Model file for the job. Use its own axes, mm. Face numbers are marked on the shaded views. A direction names the side the tool comes from. Give positions to 0.01 mm unless a question says otherwise; leave off trailing zeros. Loops run counter-clockwise (first coordinate to the right, second up) from the corner with the lowest first, then second, coordinate; pieces in that order, holes last. Notation, with made-up numbers: M 64,-3 L 116,-3 A17 cw 116,27 Z; hole C 76,55.25 d11. An arc over 180 degrees is marked long. Answer in a Markdown table with one row per item.
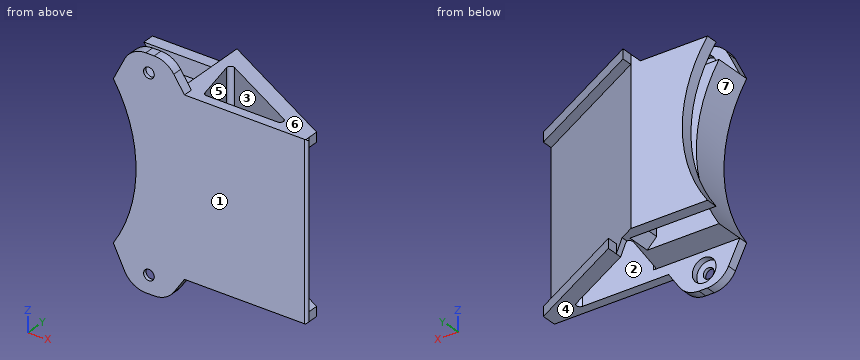
```python
from build123d import *

# Parameters (mm, degrees)
ESTRUSIONE_ESTRUSIONE1_DEPTH                         = 90
TAGLIO_ESTRUSIONE1_DEPTH                             = 60
SCHIZZO3_R                                           = 60
TAGLIO_ESTRUSIONE2_DEPTH                             = 21
ESTRUSIONE_ESTRUSIONE2_DEPTH                         = 4
FORO_LAMATO_PER_VITE_M4_A_TESTA_CILINDRI_D           = 4.5
FORO_LAMATO_PER_VITE_M4_A_TESTA_CILINDRI_DEPTH       = 8
FORO_LAMATO_PER_VITE_M4_A_TESTA_CILINDRI_CBORE_D     = 10
FORO_LAMATO_PER_VITE_M4_A_TESTA_CILINDRI_CBORE_DEPTH = 2.6
FORO_LAMATO_PER_VITE_M4_A_TESTA_CILINDRI_TIP         = 1.351936393
RACCORDO3_R                                          = 10
ESTRUSIONE_ESTRUSIONE3_DEPTH                         = 4
ESTRUSIONE_ESTRUSIONE4_DEPTH                         = 4
TAGLIO_ESTRUSIONE3_DEPTH                             = 179
SMUSSO1_SIZE                                         = 4
RACCORDO4_START                                      = -5
RACCORDO4_DEPTH                                      = 75
RACCORDO4_2_DEPTH                                    = 65
SMUSSO2_SIZE                                         = 4
SMUSSO3_SIZE                                         = 4


with BuildPart() as part:
    # Schizzo1 → Estrusione-Estrusione1 (new body)
    with BuildSketch(Plane.XY):
        Polygon((-115, 26), (0, 26), (0, 16), (-45, 16), (-45, 0), (58.302520426, 0), (0, 31), (-115, 31), align=None)
    extrude(amount=ESTRUSIONE_ESTRUSIONE1_DEPTH)

    # Schizzo2 → Taglio-Estrusione1 (cut)
    with BuildSketch(Plane(origin=(0, 31, 0), x_dir=(1, 0, 0), z_dir=(0, 1, 0))):
        with BuildLine():
            Line((-32.326881201, -65), (58.302520426, -65))
            Line((58.302520426, -65), (58.302520426, -90))
            Line((58.302520426, -90), (-115, -90))
            Line((-115, -90), (-115, 0))
            Line((-115, 0), (-32.326881201, 0))
            ThreePointArc((-32.326881201, 0), (-21.697479574, -32.5), (-32.326881201, -65))
        make_face()
    extrude(amount=-TAGLIO_ESTRUSIONE1_DEPTH, mode=Mode.SUBTRACT)

    # Schizzo3 → Taglio-Estrusione2 (cut)
    with BuildSketch(Plane.XZ):
        with Locations((-76.697479574, 32.5)):
            Circle(SCHIZZO3_R)
    extrude(amount=-TAGLIO_ESTRUSIONE2_DEPTH, mode=Mode.SUBTRACT)

    # Schizzo4 → Estrusione-Estrusione2 (add)
    with BuildSketch(Plane.XZ):
        Polygon((-26.26187707, 65), (-18.76187707, 80), (-3.76187707, 80), (3.73812293, 69), (3.73812293, 65), align=None)
        Polygon((-26.26187707, 0), (-18.76187707, -15), (-3.76187707, -15), (3.73812293, -4), (3.73812293, 0), align=None)
    extrude(amount=-ESTRUSIONE_ESTRUSIONE2_DEPTH)

    # Foro lamato per Vite M4 a testa cilindrica piana-1
    with Locations(Plane(origin=(-11.26187707, 4, 72.5), x_dir=(0, 0, 1), z_dir=(0, 1, 0))):
        with Locations((0, 0), (-80, 0)):
            CounterBoreHole(FORO_LAMATO_PER_VITE_M4_A_TESTA_CILINDRI_D / 2, FORO_LAMATO_PER_VITE_M4_A_TESTA_CILINDRI_CBORE_D / 2, FORO_LAMATO_PER_VITE_M4_A_TESTA_CILINDRI_CBORE_DEPTH, depth=FORO_LAMATO_PER_VITE_M4_A_TESTA_CILINDRI_DEPTH)
            with Locations((0, 0, -(FORO_LAMATO_PER_VITE_M4_A_TESTA_CILINDRI_DEPTH + FORO_LAMATO_PER_VITE_M4_A_TESTA_CILINDRI_TIP / 2))):  # 118° drill point
                Cone(0, FORO_LAMATO_PER_VITE_M4_A_TESTA_CILINDRI_D / 2, FORO_LAMATO_PER_VITE_M4_A_TESTA_CILINDRI_TIP, mode=Mode.SUBTRACT)

    # Raccordo3
    raccordo3_edges = [part.edges().sort_by_distance(p)[0] for p in [
        (-18.76187707, 2, 80),
        (-3.76187707, 2, 80),
        (-3.76187707, 2, -15),
        (-18.76187707, 2, -15),
    ]]
    fillet(raccordo3_edges, radius=RACCORDO3_R)

    # Schizzo9 → Estrusione-Estrusione3 (add)
    with BuildSketch(Plane.XY.offset(65)):
        Polygon((3.73812293, 0), (3.73812293, 4), (0, 4), (0, 35.530280203), (54.802520426, 6.391263214), (54.802520426, 0), align=None)
    extrude(amount=ESTRUSIONE_ESTRUSIONE3_DEPTH)

    # Schizzo10 → Estrusione-Estrusione4 (add)
    with BuildSketch(Plane(origin=(0, 0, 0), x_dir=(-1, 0, 0), z_dir=(0, 0, -1))):
        Polygon((-54.802520426, 0), (-54.802520426, 6.391263214), (-10, 30.213185886), (-10, 4), (-3.73812293, 4), (-3.73812293, 0), align=None)
    extrude(amount=ESTRUSIONE_ESTRUSIONE4_DEPTH)

    # Schizzo6 → Taglio-Estrusione3 (cut)
    with BuildSketch(Plane.XY.offset(69)):
        with BuildLine():
            Line((6.704207344, 24.902542066), (40.704207344, 6.824421389))
            ThreePointArc((40.704207344, 6.824421389), (41.455443589, 5.137117157), (40, 4))
            Line((40, 4), (10, 4))
            ThreePointArc((10, 4), (9.06087354, 4.330366941), (8.535422195, 5.175944678))
            Line((8.535422195, 5.175944678), (4.535422195, 23.254065354))
            ThreePointArc((4.535422195, 23.254065354), (5.092305295, 24.772310914), (6.704207344, 24.902542066))
        make_face()
    extrude(amount=-TAGLIO_ESTRUSIONE3_DEPTH, mode=Mode.SUBTRACT)

    # Smusso1
    # the kernel refuses this chamfer: 4 mm, written as the material it adds along each edge
    with BuildSketch(Plane(origin=(0, 15.713268048, 65), x_dir=(-1, 0, 0), z_dir=(0, 1, 0))) as smusso1_piece_1_section:
        Polygon((SMUSSO1_SIZE, 0), (0, SMUSSO1_SIZE), (0, 0), align=None)
    smusso1_piece_1 = extrude(amount=25.573463904, mode=Mode.PRIVATE)
    smusso1_piece_1 = split(smusso1_piece_1, bisect_by=Plane(origin=(0, 16, 65), z_dir=(0, -1, 0)), keep=Keep.TOP, mode=Mode.PRIVATE)
    add(smusso1_piece_1)
    with BuildSketch(Plane(origin=(0, 26, 65), x_dir=(-1, 0, 0), z_dir=(0, 1, 0))) as smusso1_piece_2:
        Polygon((SMUSSO1_SIZE, 0), (0, SMUSSO1_SIZE), (0, 0), align=None)
    extrude(amount=5)
    with BuildSketch(Plane(origin=(0, 4, 65), x_dir=(0, 0, 1), z_dir=(0, 1, 0))) as smusso1_piece_3:
        Polygon((SMUSSO1_SIZE, 0), (0, -SMUSSO1_SIZE), (0, 0), align=None)
    extrude(amount=12)
    with BuildSketch(Plane(origin=(0, -6.286731952, 65), x_dir=(0, 0, 1), z_dir=(0, 1, 0))) as smusso1_piece_4_section:
        Polygon((SMUSSO1_SIZE, 0), (0, -SMUSSO1_SIZE), (0, 0), align=None)
    smusso1_piece_4 = extrude(amount=32.573463904, mode=Mode.PRIVATE)
    smusso1_piece_4 = split(smusso1_piece_4, bisect_by=Plane(origin=(0, 26, 65), z_dir=(0, 1, 0)), keep=Keep.TOP, mode=Mode.PRIVATE)
    add(smusso1_piece_4)
    # the kernel refuses this chamfer: 4 mm, written as the material it takes off along each edge
    with BuildSketch(Plane(origin=(0, 26, 0), x_dir=(1, 0, 0), z_dir=(0, -1, 0))) as smusso1_2_piece_1:
        Polygon((SMUSSO1_SIZE, 0), (0, SMUSSO1_SIZE), (0, 0), align=None)
    extrude(amount=10, mode=Mode.SUBTRACT)

    # Raccordo4: read off the stored shape, not the designer's step
    # Raccordo4 outline → Raccordo4 (cut)
    with BuildSketch(Plane.XY.offset(RACCORDO4_START)):
        with BuildLine():
            Line((54.291739492, 0), (58.302520426, 0))
            Line((58.302520426, 0), (54.802520426, 1.860983011))
            Line((54.802520426, 1.860983011), (54.802520426, 1.859710904))
            ThreePointArc((54.802520426, 1.859710904), (55.25602962, 0.735151839), (54.291739492, 0))
        make_face()
    extrude(amount=RACCORDO4_DEPTH, mode=Mode.SUBTRACT)

    # Raccordo4 2 outline → Raccordo4 2 (cut)
    with BuildSketch(Plane.XY):
        with BuildLine():
            ThreePointArc((54.761211055, 1.882947593), (54.782003426, 1.871574022), (54.802520426, 1.859710904))
            Line((54.802520426, 1.859710904), (54.802520426, 1.860983011))
            Line((54.802520426, 1.860983011), (54.761211055, 1.882947593))
        make_face()
    extrude(amount=RACCORDO4_2_DEPTH, mode=Mode.SUBTRACT)

    # Smusso2
    # the kernel refuses this chamfer: 4 mm, written as the material it adds along each edge
    with BuildSketch(Plane(origin=(54.802520426, 12.146442856, 65), x_dir=(0, 0, 1), z_dir=(0, -1, 0))) as smusso2_piece_1_section:
        Polygon((SMUSSO2_SIZE, 0), (0, -SMUSSO2_SIZE), (0, 0), align=None)
    smusso2_piece_1 = extrude(amount=22.292885711, mode=Mode.PRIVATE)
    smusso2_piece_1 = smusso2_piece_1 & Plane(origin=(54.291739491, 1, 65), x_dir=(0.5107809344553311, 0.8597109031511343, 0), z_dir=(0, 0, -1)) * Cylinder(1, 61, mode=Mode.PRIVATE)
    add(smusso2_piece_1)
    # the kernel refuses this chamfer: 4 mm, written as the material it adds along each edge
    with BuildSketch(Plane(origin=(54.802520426, -10.146442855, 0), x_dir=(0, 0, -1), z_dir=(0, 1, 0))) as smusso2_2_piece_1_section:
        Polygon((SMUSSO2_SIZE, 0), (0, -SMUSSO2_SIZE), (0, 0), align=None)
    smusso2_2_piece_1 = extrude(amount=22.292885711, mode=Mode.PRIVATE)
    smusso2_2_piece_1 = smusso2_2_piece_1 & Plane(origin=(54.291739491, 1, 0), x_dir=(0.5107809344553311, 0.8597109031511343, 0), z_dir=(0, 0, -1)) * Cylinder(1, 61, mode=Mode.PRIVATE)
    add(smusso2_2_piece_1)

    # Smusso3
    smusso3_edges = [part.edges().sort_by_distance(p)[0] for p in [
        (10, 24.416521855, 0),
    ]]
    chamfer(smusso3_edges, length=SMUSSO3_SIZE - 0.0001)  # a hair under: the kernel refuses the full size


solid = part.part
```
(1) Wall check: L1, parallel to Y at x = -12, z = 20; L2, parallel to Z at x = 18, y = 24.5; L3, parallel to X at y = 0.7, z = -7.5. Give the ranges that are in metal, low to high.
Established:
| item | result |
|---|---|
| L1 | y = 0 to 16, 26 to 31 |
| L2 | z = -4 to 0, 65 to 69 |
| L3 | x = -22.51 to -13.51, -9.01 to 1.35 |
(2) Mould opens along X. For the marked faces 5, 6 and 7 say: pulls with the +X half, pulls with the -X half, needs draft (parallel to the pull), parting line crosses it, or undercut.
Established:
| item | result |
|---|---|
| face 5 | undercut |
| face 6 | needs draft |
| face 7 | pulls with the -X half |
(3) Flat gauge pins, fed straight in: P1, Ø1.2, axis at y = 26.5, z = -1.5, coming from the -X side; P2, Ø4.5, axis at x = -16.5, z = 72, coming from the +Y side; P3, Ø6, axis at x = -20, y = 7.5, coming from the +Z side. Where does each tip first touch, or does it go through?
Established:
| item | result |
|---|---|
| P1 | stops at x = 6.9 |
| P2 | stops at y = 4 |
| P3 | stops at z = 65 |
(4) Saw through at A-A, the plane x = 21. Give the cut face in (y, z).
Established:
| item | result |
|---|---|
| outline | M 0,-4 L 4,-4 L 4,69 L 0,69 Z; M 17.3,-4 L 24.36,-4 L 24.36,0 L 19.83,0 L 19.83,65 L 24.36,65 L 24.36,69 L 17.3,69 Z |
(5) Saw through at C-C, the plane y = 9.5. Give the cut face in (x, z), and give its area (3 significant figures).
Established:
| item | result |
|---|---|
| outline | M -26.26,0 L 7.58,0 L 7.58,69 L 0,69 L -4,65 L -26.26,65 A60 cw Z; M 35.67,-4 L 48.96,-4 L 48.96,0 L 40.44,0 L 40.44,65 L 48.96,65 L 48.96,69 L 35.67,69 Z |
| area | 2,230 mm2 |
(6) Saw through at D-D, the plane z = 22. Give the cut face in (x, y), and give its area (3 significant figures).
Established:
| item | result |
|---|---|
| outline | M -22.71,26 L 0,26 L 0,16 L -17.62,16 L -17.62,0 L 54.29,0 A1 ccw 54.76,1.88 L 0,31 L -22.71,31 Z; hole M 4.54,23.25 L 8.54,5.18 A1.5 ccw 10,4 L 40,4 A1.5 ccw 40.7,6.82 L 6.7,24.9 A1.5 ccw Z |
| area | 888 mm2 |
(7) Which spindle directions (+Z, -Z, +X, -X, +Y, -Y) get a long thin tool onto all of the face, cutting with end or side? Do the marked faces 1, 2, 3 and 4. Say none if no direction does.
Established:
| item | result |
|---|---|
| face 1 | +Z, -Z, +X, -X, -Y |
| face 2 | -Z |
| face 3 | +Z, -Z |
| face 4 | -Z, +X, +Y, -Y |
(8) Saw through at B-B, the plane z = 72.5. Give the cut face in (x, y).
Established:
| item | result |
|---|---|
| outline | M -22.51,0 L -13.51,0 L -13.51,1.4 L -16.26,1.4 L -16.26,4 L -22.51,4 Z; M -9.01,0 L 1.35,0 L 1.35,4 L -6.26,4 L -6.26,1.4 L -9.01,1.4 Z |
